Autodesk Inventor part; units mm, degrees
ref_plane "YZ Plane" through (0, 0, 0) normal (1, 0, 0) x (0, 1, 0)
ref_plane "XZ Plane" through (0, 0, 0) normal (0, 1, 0) x (-1, 0, 0)
ref_plane "XY Plane" through (0, 0, 0) normal (0, 0, 1) x (1, 0, 0)
sketch "스케치2" plane through (0, 0, 0) normal (0, 1, 0) x (-1, 0, 0)
  line L0 (12.4336, 17.7711) -> (-13.7162, 17.7711)
  line L1 (-13.7162, 17.7711) -> (-13.7162, -22.5294)
  line L2 (-13.7162, -22.5294) -> (12.4336, -22.5294)
  line L3 (12.4336, -22.5294) -> (12.4336, 17.7711)
  point P0 (0, 0)
extrude "돌출1" add sketch "스케치2" along normal blind 10
sketch "스케치3" plane through (0, 10, 0) normal (0, 1, 0) x (1, 0, 0)
  line L0 (-12.4336, 22.5294) -> (-12.4336, -17.7711)
  line L1 (-12.4336, -17.7711) -> (-7.0874, -17.7711)
  line L2 (-7.0874, -17.7711) -> (-7.0874, -9.3549)
  line L3 (-7.0874, -9.3549) -> (-12.4336, -9.3549)
  line L4 (-12.4336, -9.3549) -> (-12.4336, -17.7711)
  point P0 (0, 0)
extrude "돌출2" add sketch "스케치3" along normal blind 10
sketch "스케치4" plane through (0, 10, 0) normal (0, 1, 0) x (1, 0, 0)
  line L0 (-12.4336, -17.7711) -> (13.7162, -17.7711)
  line L1 (13.7162, -17.7711) -> (8.3702, -17.7711)
  line L2 (8.3702, -17.7711) -> (8.3702, -9.3551)
  line L3 (8.3702, -9.3551) -> (13.7162, -9.3551)
  line L4 (13.7162, -9.3551) -> (13.7162, -17.7711)
  point P0 (0, 0)
  dimension "d4" = 5.346
  dimension "d5" = 8.416
extrude "돌출3" add sketch "스케치4" along normal blind 8.416
sketch "스케치5" plane through (-12.4336, 0, 17.7711) normal (0, 0, 1) x (1, 0, 0)
  line L0 (5.3461, 10) -> (20.8038, 10)
  line L1 (0, 0) -> (26.1498, 0)
  line L2 (5.3461, 10) -> (20.8037, 10)
  line L3 (20.8037, 10) -> (20.8037, 0)
  line L4 (20.8037, 0) -> (5.3461, 0)
  line L5 (5.3461, 0) -> (5.3461, 10)
  point P0 (12.4336, 0)
  dimension "d8" = 26.1498
sketch "스케치6" plane through (0, 20, 0) normal (0, 1, 0) x (1, 0, 0)
  point P0 (0, 0)
extrude "돌출4" cut sketch "스케치5" against normal blind 8.416
equation "\"d6\" = d5"
properties part number "공부용"
Design review of the part built by this model. Coordinates are the model's own, in mm. A direction names the side the tool comes from. Round coordinates to 2 decimals unless told otherwise and drop trailing zeros. Write each loop counter-clockwise with the first axis right and the second up, starting at its lowest first coordinate (ties: lowest second). Pieces come first, ordered by that corner, then holes. Notation, with made-up numbers: (-2, 18) - (57, 18) arc R28 cw to (57, 48) - close; hole circle Ø6 at (67.5, -28). An arc over 180 degrees is marked (long way). Use a Markdown table: item, result. Add a question column.
1. Clearance check with flat-ended pins moving along their axes: pin 1 (1.6 mm diameter, centred on x = 11.5, z = 14, fed in from +Y); pin 2 (6 mm diameter, centred on x = -9.5, y = 15.5, fed in from -Z). State where each tip first meets the part, or that it passes through.
2. We need section D-D (y = 6). State the section outline as (x, z) points, then the cut area to 3 significant figures.
3. We need section C-C (x = 7.75). State the section outline as (y, z) points, then the cut area to 3 significant figures.
4. Mouldability with a two-part tool opening along X and no side actions: class faces 1 (the face through (-12.434, 8, 2)), 2 (the face through (-7.087, 15, 14)), 3 (the face through (11, 14, 9.355)) as +X half, -X half, draft (parallel to the pull), parting line (faces both ways), or undercut.
5. We need section A-A (y = 12.25). State the section outline as (x, z) points, then the cut area to 3 significant figures.
6. We need section B-B (z = -7). State the section outline as (x, y) points.
7. Wall thickness on probe 1 along X at (y, z) = (3.5, 9.5); probe 2 along Y at (x, z) = (10, -7); probe 3 along Z at (x, y) = (-3.5, 7.75): over which ranges is each line inside the solid? List them lowest first.
8. For faces 4 (the face through (1, 0, -2)), 5 (the face through (1, 5, 9.355)), 6 (the face through (11, 18.416, 14)), 7 (the face through (1, 10, -6)), list the 3-axis set-ups (+Z, -Z, +X, -X, +Y, -Y) from which the entire face can be reached by the end or side of a thin tool; tool diameter is ignored.
Output:
| question | item | result |
|---|---|---|
| 1 | pin 1 | stops at y = 18.42 |
| 1 | pin 2 | stops at z = 9.35 |
| 2 | outline | (-12.43, -22.53) - (13.72, -22.53) - (13.72, 17.77) - (8.37, 17.77) - (8.37, 9.36) - (-7.09, 9.36) - (-7.09, 17.77) - (-12.43, 17.77) - close |
| 2 | area | 924 mm2 |
| 3 | outline | (0, -22.53) - (10, -22.53) - (10, 9.36) - (0, 9.36) - close |
| 3 | area | 319 mm2 |
| 4 | face 1 | -X half |
| 4 | face 2 | undercut |
| 4 | face 3 | draft |
| 5 | outline | (-12.43, 9.35) - (-7.09, 9.35) - (-7.09, 17.77) - (-12.43, 17.77) - close; (8.37, 9.36) - (13.72, 9.36) - (13.72, 17.77) - (8.37, 17.77) - close |
| 5 | area | 90.0 mm2 |
| 6 | outline | (-12.43, 0) - (13.72, 0) - (13.72, 10) - (-12.43, 10) - close |
| 7 | probe 1 | x = -12.43 to -7.09, 8.37 to 13.72 |
| 7 | probe 2 | y = 0 to 10 |
| 7 | probe 3 | z = -22.53 to 9.36 |
| 8 | face 4 | +Z, -Z, +X, -X, -Y |
| 8 | face 5 | +Z, +Y, -Y |
| 8 | face 6 | +Z, -Z, +X, +Y |
| 8 | face 7 | -Z, +X, -X, +Y |
